from build123d import *

# Parameters (mm, degrees)
BOSS_EXTRUDE1_DEPTH = 1.5
BOSS_EXTRUDE2_DEPTH = 9
BOSS_EXTRUDE3_DEPTH = 1
SKETCH4_R           = 5
SKETCH4_R_2         = 4
BOSS_EXTRUDE4_DEPTH = 10
FILLET1_R           = 5


with BuildPart() as part:
    # Sketch1 → Boss-Extrude1 (new body)
    with BuildSketch(Plane(origin=(0, 0, 0), x_dir=(0, 1, 0), z_dir=(0, 0, 1))):
        Polygon((-62.5, -42.5), (-62.5, 42.5), (55.428932188, 42.5), (62.5, 35.428932188), (62.5, -35.428932188), (55.428932188, -42.5), align=None)
        Polygon((54.050252532, 40), (59, 35.050252532), (59, -35.050252532), (54.050252532, -40), (-59, -40), (-59, 40), align=None, mode=Mode.SUBTRACT)
    extrude(amount=BOSS_EXTRUDE1_DEPTH)

    # Sketch2 → Boss-Extrude2 (add)
    with BuildSketch(Plane(origin=(0, 0, 0), x_dir=(0, 1, 0), z_dir=(0, 0, 1))):
        Polygon((-63.5, 43.5), (-63.5, -43.5), (55.721825407, -43.5), (63.5, -35.721825407), (63.5, 35.721825407), (55.721825407, 43.5), align=None)
        Polygon((-62.5, -42.5), (55.428932188, -42.5), (62.5, -35.428932188), (62.5, 35.428932188), (55.428932188, 42.5), (-62.5, 42.5), align=None, mode=Mode.SUBTRACT)
    extrude(amount=BOSS_EXTRUDE2_DEPTH)

    # Sketch3 → Boss-Extrude3 (add)
    with BuildSketch(Plane(origin=(0, 0, 0), x_dir=(0, 1, 0), z_dir=(0, 0, 1))):
        Polygon((63.5, 35.721825407), (55.721825407, 43.5), (-63.5, 43.5), (-63.5, -43.5), (55.721825407, -43.5), (63.5, -35.721825407), align=None)
    extrude(amount=-BOSS_EXTRUDE3_DEPTH)

    # Sketch4 → Boss-Extrude4 (add)
    with BuildSketch(Plane(origin=(0, 0, -1), x_dir=(1, 0, 0), z_dir=(0, 0, -1))):
        Circle(SKETCH4_R)
        with Locations(Location((0, 0, 0), (0, 0, 180))):
            Circle(SKETCH4_R_2, mode=Mode.SUBTRACT)
    extrude(amount=BOSS_EXTRUDE4_DEPTH)

    # Fillet1
    fillet1_edges = [part.edges().sort_by_distance(p)[0] for p in [
        (-5, 0, -1),
    ]]
    fillet(fillet1_edges, radius=FILLET1_R)


solid = part.part
The listing builds one solid part. Answer for the finished solid, in the listing's coordinates (mm). A direction names the side the tool comes from. Coordinates: 2 decimals unless noted, no trailing zeros. Write each loop counter-clockwise with the first axis right and the second up, starting at its lowest first coordinate (ties: lowest second). Pieces come first, ordered by that corner, then holes. Notation, with made-up numbers: (2.25, -25.75) - (53.25, -25.75) arc R11 ccw to (53.25, -20.75) - close; hole circle Ø3 at (65.5, 82.5). An arc over 180 degrees is marked (long way). Put each result on its own line as item: value.
1. A tool of negligible diameter and unlimited length cuts with its end or side. For faces 1 (the face through (-42.5, -3, 5)), 2 (the face through (1, 63.5, 4)), 3 (the face through (0.867, -3.905, -5.93)), from which of +Z, -Z, +X, -X, +Y, -Y can it reach the whole face along a straight path? Write none if from no direction.
Answer sheet:
face 1: +Z
face 2: +Z, -Z, +X, -X, +Y
face 3: -Z
2. The part is cut by section C-C on y = 0. Give the vertices of the cut face in (x, z).
Answer sheet:
outline: (-43.5, -1) - (-10, -1) arc R5 cw to (-5, -6) - (-5, -11) - (-4, -11) - (-4, -1) - (4, -1) - (4, -11) - (5, -11) - (5, -6) arc R5 cw to (10, -1) - (43.5, -1) - (43.5, 9) - (42.5, 9) - (42.5, 1.5) - (40, 1.5) - (40, 0) - (-40, 0) - (-40, 1.5) - (-42.5, 1.5) - (-42.5, 9) - (-43.5, 9) - close
3. Find the intervals of material crossed by line 1 along Y through (x, z) = (0, -6); line 2 along Y through (x, z) = (-20, 0.5); line 3 along Z through (x, y) = (-9.5, 4), in increasing order. Write a range as from..to.
Answer sheet:
line 1: y = -5..-4, 4..5
line 2: y = -63.5..-59, 59..63.5
line 3: z = -1..0
4. The part is cut by section D-D on z = -2.75. Give the vertices of the cut face in (x, y), plus the area to 3 significant figures.
Answer sheet:
outline: circle Ø12.4 at (0, 0); hole circle Ø8 at (0, 0)
area: 70.5 mm^2
5. Flat-ended cylindrical pins translate along their axes: pin 1 Ø6 at (x, y) = (10.5, 11.5) entering from -Z; pin 2 Ø4 at (x, y) = (7.5, 18.5) entering from +Z. Find the tip coordinate at first contact, or state that the pin passes through.
Answer sheet:
pin 1: stops at z = -1
pin 2: stops at z = 0
6. The part is cut by section A-A on z = 3. Give the vertices of the cut face in (x, y), plus the area to 4 significant figures.
Answer sheet:
outline: (-43.5, -63.5) - (43.5, -63.5) - (43.5, 55.72) - (35.72, 63.5) - (-35.72, 63.5) - (-43.5, 55.72) - close; hole (-42.5, -62.5) - (42.5, -62.5) - (42.5, 55.43) - (35.43, 62.5) - (-35.43, 62.5) - (-42.5, 55.43) - close
area: 413.5 mm^2
7. Determine the mould class of faces 4 (the face through (-43.5, -3, 4)), 5 (the face through (-1, -63.5, 4)), 6 (the face through (42.5, -4, 5)), 7 (the face through (-39.556, 59.665, 4.07)) for opening direction Y: pulls with the +Y half, pulls with the -Y half, needs draft (parallel to the pull), parting line crosses it, or undercut.
Answer sheet:
face 4: needs draft
face 5: pulls with the -Y half
face 6: undercut
face 7: pulls with the +Y half
8. The part is cut by section B-B on x = 0. Give the vertices of the cut face in (y, z), plus the area to 3 significant figures.
Answer sheet:
outline: (-63.5, -1) - (-10, -1) arc R5 cw to (-5, -6) - (-5, -11) - (-4, -11) - (-4, -1) - (4, -1) - (4, -11) - (5, -11) - (5, -6) arc R5 cw to (10, -1) - (63.5, -1) - (63.5, 9) - (62.5, 9) - (62.5, 1.5) - (59, 1.5) - (59, 0) - (-59, 0) - (-59, 1.5) - (-62.5, 1.5) - (-62.5, 9) - (-63.5, 9) - close
area: 186 mm^2
